The listing builds one solid part. Answer for the finished solid, in the listing's coordinates (mm). Round coordinates to 2 decimals unless told otherwise and drop trailing zeros. Order: outer loops, then holes, each group sorted by start corner. A loop starts at its lowest first (then second) coordinate and runs counter-clockwise, first axis right, second up. Notation, with made-up numbers: M 80.25,51 L 122.25,51 A24 cw 122.25,68 Z; hole C 48,29 d2. An arc over 180 degrees is marked long. Put each result on its own line as item: value. Start each with the question number.
1. The part is cut by section B-B (z = -9). Give the vertices of the cut face in (x, y).
2. The part is cut by section A-A (z = -4). Give the vertices of the cut face in (x, y).
3. Consider line 1 (Y direction, x = 0.5, z = -0.25); line 2 (X direction, y = -2.75, z = -1.75); line 3 (Y direction, x = 2, z = -6.75). Determine where each line is inside the solid, lowest interval first.
4. The part is cut by section C-C (z = -0.75). Give the vertices of the cut face in (x, y), then the cut area to 3 significant figures.
5. Each of these flat-tipped pins is pushed along its axis until it touches: pin 1 Ø4 at (x, z) = (5, -5) entering from +Y; pin 2 Ø4 at (y, z) = (7.5, -3) entering from +X; pin 3 Ø5 at (x, y) = (-1, 0.5) entering from +Z. Where does it stop, or does it pass through?
6. The mould has two halves that part along Y. Classify faces 1 (the face through (7.84, 4.55, -0.27)), 2 (the face through (-1.08, -4.84, -4.81)), 3 (the face through (7.86, -4.51, -9.51)): +Y half, -Y half, draft (parallel to the pull), parting line (faces both ways), or undercut.
from build123d import *

# Parameters (mm, degrees)
BASENUTSKE_R  = 4.96062
BASENUT_DEPTH = 9.779


with BuildPart() as part:
    # BaseNutSke → BaseNut (new body)
    with BuildSketch(Plane.XY):
        Polygon((8.7376, 5.044655712), (8.7376, -5.044655712), (0, -10.089311424), (-8.7376, -5.044655712), (-8.7376, 5.044655712), (0, 10.089311424), align=None)
        Circle(BASENUTSKE_R, mode=Mode.SUBTRACT)
    extrude(amount=-BASENUT_DEPTH)

    # Sketch3 → Double-Chamfer (revolve, cut)
    with BuildSketch(Plane(origin=(0, 0, 0), x_dir=(0, 0, -1), z_dir=(1, 0, 0))):
        Polygon((9.779, 8.7376), (8.66775, 10.089311424), (8.66775, 22.789311424), (22.479, 22.789311424), (22.479, 8.7376), align=None)
        Polygon((1.11125, 22.789311424), (-12.7, 22.789311424), (-12.7, 8.7376), (0, 8.7376), (1.11125, 10.089311424), align=None)
    revolve(axis=Axis((0, 0, 0), (0, 0, -1)), mode=Mode.SUBTRACT)

    # Sketch5 → EndChamfer (revolve, cut)
    with BuildSketch(Plane(origin=(0, 0, 0), x_dir=(0, 0, -1), z_dir=(1, 0, 0)), mode=Mode.PRIVATE) as endchamfer_sk:
        Polygon((9.7536, 5.55625), (9.294828922, 4.901057), (9.8044, 4.901057), (9.8044, 5.55625), align=None)
        Polygon((-0.0508, 5.55625), (0, 5.55625), (0.458771078, 4.901057), (-0.0508, 4.901057), align=None)
    revolve(endchamfer_sk.sketch.rotate(Axis((0, 0, -25.037505729), (0, 0, -1)), 90), axis=Axis((0, 0, -25.037505729), (0, 0, -1)), mode=Mode.SUBTRACT)


solid = part.part
Resolved:
1. outline: M -8.74,-4.18 A9.69 ccw -7.99,-5.48 L -0.75,-9.66 A9.69 ccw 0.75,-9.66 L 7.99,-5.48 A9.69 ccw 8.74,-4.18 L 8.74,4.18 A9.69 ccw 7.99,5.48 L 0.75,9.66 A9.69 ccw -0.75,9.66 L -7.99,5.48 A9.69 ccw -8.74,4.18 Z; hole C 0,0 d9.92
2. outline: M -8.74,-5.04 L 0,-10.09 L 8.74,-5.04 L 8.74,5.04 L 0,10.09 L -8.74,5.04 Z; hole C 0,0 d9.92
3. line 1: -9.03 to -5.18, 5.18 to 9.03
3. line 2: -8.74 to -4.13, 4.13 to 8.74
3. line 3: -8.93 to -4.54, 4.54 to 8.93
4. outline: M -8.74,-4.1 A9.65 ccw -7.92,-5.52 L -0.82,-9.61 A9.65 ccw 0.82,-9.61 L 7.92,-5.52 A9.65 ccw 8.74,-4.1 L 8.74,4.1 A9.65 ccw 7.92,5.52 L 0.82,9.61 A9.65 ccw -0.82,9.61 L -7.92,5.52 A9.65 ccw -8.74,4.1 Z; hole C 0,0 d9.92
4. area: 185 mm2
5. pin 1: y = 8.36
5. pin 2: x = 7.95
5. pin 3: through
6. face 1: +Y half
6. face 2: undercut
6. face 3: -Y half
